Geometry check sheet. Reference: drawing and pictorial views, mm from the part's lowest x, y, z. A direction names the side the tool comes from. Give positions to 0.01 mm unless a question says otherwise; leave off trailing zeros. Loops run counter-clockwise (first coordinate to the right, second up) from the corner with the lowest first, then second, coordinate; pieces in that order, holes last. Notation, with made-up numbers: M -19,33 L 1,33 A26 ccw 1,54 Z; hole C -13.75,14.5 d3. An arc over 180 degrees is marked long. Use CSV: the item, a comma, the result in double quotes.
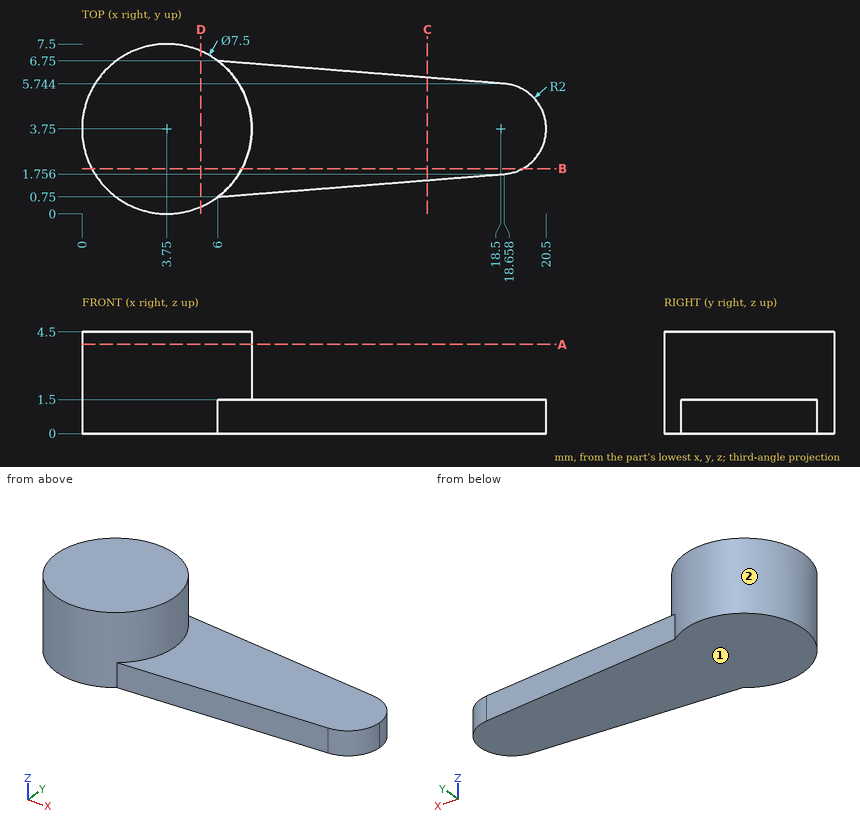
(1) Section check A-A on z = 3.95. Record the cut outline in (x, y).
Calculated:
outline,"C 3.75,3.75 d7.5"
(2) Section check B-B on y = 2. Record the cut outline in (x, z).
Calculated:
outline,"M 0.43,0 L 19.47,0 L 19.47,1.5 L 7.07,1.5 L 7.07,4.5 L 0.43,4.5 Z"
(3) Scan lines: L1, parallel to Z at x = 14, y = 3.5; L2, parallel to X at y = 6, z = 3.35; L3, parallel to X at y = 0.75, z = 1.6. Record each from-to range of solid material in increasing order. Write a range as from..to.
Calculated:
L1,"z = 0..1.5"
L2,"x = 0.75..6.75"
L3,"x = 1.5..6"
(4) Section check D-D on x = 5.25. Record the cut outline in (y, z).
Calculated:
outline,"M 0.31,0 L 7.19,0 L 7.19,4.5 L 0.31,4.5 Z"
(5) Depth check by flat-ended pin: pin 1 Ø3 at (x, y) = (13, 4) entering from +Z; pin 2 Ø1.5 at (y, z) = (4.5, 3.5) entering from +X. Enter the tip coordinate at first touch or a pass-through.
Calculated:
pin 1,"stops at z = 1.5"
pin 2,"stops at x = 7.5"
(6) Section check C-C on x = 15.25. Record the cut outline in (y, z) (1 decimal).
Calculated:
outline,"M 1.5,0 L 6,0 L 6,1.5 L 1.5,1.5 Z"
(7) Tool access check on the marked faces 1 and 2. Record the directions out of +Z, -Z, +X, -X, +Y, -Y that give a thin tool (end or side, any length) a straight path to the whole face; none if there is none.
Calculated:
face 1,"-Z, +X, -X, +Y, -Y"
face 2,"+Z"
